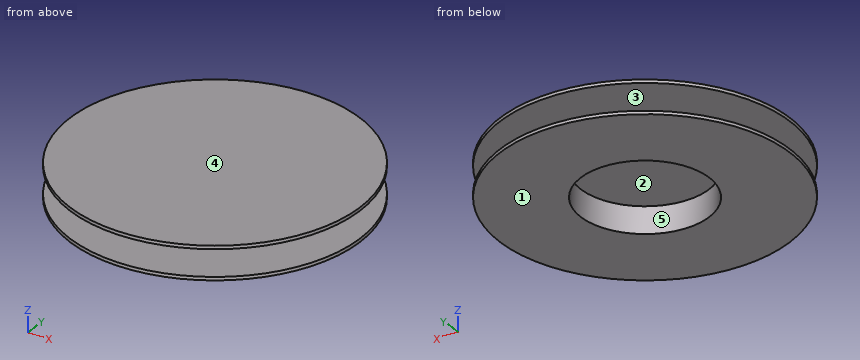
```python
from build123d import *

# Parameters (mm, degrees)
F0_R     = 11.7
F0_R_2   = 9.6
F1_DEPTH = 5
F0_R_3   = 21.7
F2_DEPTH = 0.5
F3_START = 4.5
F3_DEPTH = 0.5
F4_START = 4
F4_DEPTH = 1


with BuildPart() as f1:
    # F0 (on Top) → F1 (new body)
    with BuildSketch(Plane.XY):
        Circle(F0_R)
        Circle(F0_R_2, mode=Mode.SUBTRACT)
    extrude(amount=F1_DEPTH)

    # F0 (on Top) → F2 (join)
    with BuildSketch(Plane.XY):
        Circle(F0_R_3)
        Circle(F0_R, mode=Mode.SUBTRACT)
    extrude(amount=F2_DEPTH)

    # F0 (on Top) → F3 (join)
    with BuildSketch(Plane.XY.offset(F3_START)):
        Circle(F0_R_3)
        Circle(F0_R, mode=Mode.SUBTRACT)
    extrude(amount=F3_DEPTH)

    # F0 (on Top) → F4 (join)
    with BuildSketch(Plane.XY.offset(F4_START)):
        Circle(F0_R_2)
    extrude(amount=F4_DEPTH)


solid = f1.part
```
Geometry: final body of the model. Coordinates: model frame, mm. Face numbers are marked on the shaded views. A direction names the side the tool comes from. Round coordinates to 2 decimals unless told otherwise and drop trailing zeros. Order: outer loops, then holes, each group sorted by start corner. A loop starts at its lowest first (then second) coordinate and runs counter-clockwise, first axis right, second up. Notation, with made-up numbers: (59.25, 10) -> (71.25, 10) arc R14 ccw to (71.25, 15) -> close; hole circle Ø7 at (-9, -5). An arc over 180 degrees is marked (long way). Use one line per item in the form item = value.
(1) Section C-C on z = 2.95. Return loops of the section in (x, y), and give its area (3 significant figures).
Results list:
outline = circle Ø23.4 at (0, 0); hole circle Ø19.2 at (0, 0)
area = 141 mm^2
(2) Draft query along Y for the marked faces 4 and 5. Return one class per face: pulls with the +Y half, pulls with the -Y half, needs draft (parallel to the pull), parting line crosses it, or undercut.
Results list:
face_4 = needs draft
face_5 = undercut
(3) First-contact query: pin 1 Ø15.5 at (x, y) = (0, 0) entering from -Z; pin 2 Ø3 at (y, z) = (10.5, 0.5) entering from +X. Flat tips, straight axial feed; report the tip coordinate or a pass-through.
Results list:
pin_1 = 4
pin_2 = 19.75
(4) Ray query, probe 1 along Z at (x, y) = (-6, -10.5); probe 2 along Y at (x, z) = (0, 2.85); probe 3 along Z at (x, y) = (-5.5, -3). Return the intervals inside material, ascending. Write a range as [from, to].
Results list:
probe_1 = [0, 0.5], [4.5, 5]
probe_2 = [-11.7, -9.6], [9.6, 11.7]
probe_3 = [4, 5]
(5) Section A-A on x = 0. Return loops of the section in (y, z).
Results list:
outline = (-21.7, 0) -> (-9.6, 0) -> (-9.6, 4) -> (9.6, 4) -> (9.6, 0) -> (21.7, 0) -> (21.7, 0.5) -> (11.7, 0.5) -> (11.7, 4.5) -> (21.7, 4.5) -> (21.7, 5) -> (-21.7, 5) -> (-21.7, 4.5) -> (-11.7, 4.5) -> (-11.7, 0.5) -> (-21.7, 0.5) -> close
(6) Access query for the marked faces 1, 2 and 3. Directions: +Z, -Z, +X, -X, +Y, -Y. A direction counts if a zero-diameter tool reaches every point of the face in a straight line with its end or side. Return the directions, or none.
Results list:
face_1 = -Z, +X, -X, +Y, -Y
face_2 = -Z
face_3 = none
